from build123d import *

# Parameters (mm, degrees)
SKETCH2_W           = 31.75
SKETCH2_H           = 25.4
BOSS_EXTRUDE1_DEPTH = 6.35
SKETCH4_R           = 1.778
SKETCH4_R_2         = 1.524
BOSS_EXTRUDE2_DEPTH = 1.905


with BuildPart() as part:
    # Sketch2 → Boss-Extrude1 (new body)
    with BuildSketch(Plane(origin=(0, 0, 0), x_dir=(1, 0, 0), z_dir=(0, 1, 0))):
        with Locations((15.875, 12.7)):
            Rectangle(SKETCH2_W, SKETCH2_H)
    extrude(amount=BOSS_EXTRUDE1_DEPTH)

    # Sketch4 → Boss-Extrude2 (add)
    with BuildSketch(Plane(origin=(0, 6.35, 0), x_dir=(1, 0, 0), z_dir=(0, 1, 0))):
        with Locations(Location((6.35, 6.35, 0), (0, 0, 90))):
            Circle(SKETCH4_R)
        with Locations(Location((6.35, 12.7, 0), (0, 0, 90))):
            Circle(SKETCH4_R)
        with Locations(Location((6.35, 19.05, 0), (0, 0, 90))):
            Circle(SKETCH4_R)
        with Locations(Location((11.43, 20.32, 0), (0, 0, 90))):
            Circle(SKETCH4_R_2)
        with Locations(Location((11.43, 15.24, 0), (0, 0, 90))):
            Circle(SKETCH4_R_2)
        with Locations(Location((11.43, 10.16, 0), (0, 0, 90))):
            Circle(SKETCH4_R_2)
        with Locations(Location((11.43, 5.08, 0), (0, 0, 90))):
            Circle(SKETCH4_R_2)
    extrude(amount=BOSS_EXTRUDE2_DEPTH)


solid = part.part
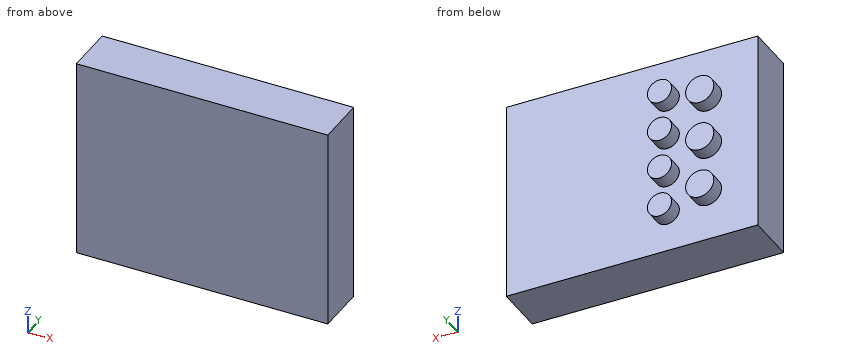
For this review, take the finished solid that the model builds, in its own axes (mm). Give positions to 0.01 mm unless a question says otherwise; leave off trailing zeros. Loops run counter-clockwise (first coordinate to the right, second up) from the corner with the lowest first, then second, coordinate; pieces in that order, holes last. Notation, with made-up numbers: M -37.75,15 L -30.75,15 A21 ccw -30.75,54 Z; hole C -37,29.5 d4. An arc over 180 degrees is marked long. Answer as a JSON object with one key per item and string values. Group by question number.
Q1. Add section A-A on z = -12.7. Give the boundary of the cut face in (x, y) (3 decimals).
Q2. Add section C-C on x = 11.43. Give the boundary of the cut face in (y, z) (3 decimals), and give its area (3 significant figures).
Q3. For probe 1 along Y at (x, z) = (13.5, -14.5), list the stretches that pass through material, from the lowest coordinate up. Write a range as [from, to].
Q4. Add section D-D on z = -7.25. Give the boundary of the cut face in (x, y) (3 decimals), and give its area (3 significant figures).
Q5. Insertion check: P1, Ø3, axis at x = 4.5, z = -16, coming from the +Y side. The pin has a flat end and moves straight along its axis. Give the tip position at first contact, or say it passes through.
Q6. Add section B-B on y = 7. Give the boundary of the cut face in (x, z).
Checked values:
{
 "1": {"outline": "M 0,0 L 31.75,0 L 31.75,6.35 L 8.128,6.35 L 8.128,8.255 L 4.572,8.255 L 4.572,6.35 L 0,6.35 Z"},
 "2": {"outline": "M 0,-25.4 L 6.35,-25.4 L 6.35,-21.844 L 8.255,-21.844 L 8.255,-18.796 L 6.35,-18.796 L 6.35,-16.764 L 8.255,-16.764 L 8.255,-13.716 L 6.35,-13.716 L 6.35,-11.684 L 8.255,-11.684 L 8.255,-8.636 L 6.35,-8.636 L 6.35,-6.604 L 8.255,-6.604 L 8.255,-3.556 L 6.35,-3.556 L 6.35,0 L 0,0 Z", "area": "185 mm²"},
 "3": {"probe 1": "[0, 6.35]"},
 "4": {"outline": "M 0,0 L 31.75,0 L 31.75,6.35 L 7.883,6.35 L 7.883,8.255 L 4.817,8.255 L 4.817,6.35 L 0,6.35 Z", "area": "207 mm²"},
 "5": {"P1": "y = 6.35"},
 "6": {"outline": "C 6.35,-19.05 d3.56; C 6.35,-12.7 d3.56; C 6.35,-6.35 d3.56; C 11.43,-20.32 d3.05; C 11.43,-15.24 d3.05; C 11.43,-10.16 d3.05; C 11.43,-5.08 d3.05"}
}
